Check sheet for the drawn part. Datum: minimum x, y, z corner. Units: mm. A direction names the side the tool comes from. Give positions to 0.01 mm unless a question says otherwise; leave off trailing zeros. Order: outer loops, then holes, each group sorted by start corner. A loop starts at its lowest first (then second) coordinate and runs counter-clockwise, first axis right, second up. Notation, with made-up numbers: (14, 25) - (37, 25) arc R22 ccw to (37, 45) - close; hole circle Ø10 at (77.5, 67). An arc over 180 degrees is marked (long way). Answer as a JSON object with one key per item and string values. Group by question number.
(1) Mould release check, pull along X, two halves, no side actions. Record for the marked faces 3, 4 and 5: +X half, -X half, draft (parallel to the pull), parting line (faces both ways), or undercut.
(2) Access from +Z, -Z, +X, -X, +Y, -Y to the whole of each face (thin tool, end or side, straight path). Record for the marked faces 1 and 2.
(3) Section check A-A (z = 6). Record the boundary of the cut face in (x, y).
(4) Section check B-B (y = 7.5). Record the boundary of the cut face in (x, z).
(5) Thickness scan on line 1 (X direction, y = 2, z = 5.75); line 2 (Z direction, x = 6.25, y = 11.5). Record the ranges inside material, lowest first.
(6) Depth check by flat-ended pin: pin 1 Ø4 at (x, y) = (5.5, 10.5) entering from -Z; pin 2 Ø0.6 at (x, z) = (0.5, 4.5) entering from +Y. Enter the tip coordinate at first touch or a pass-through.
(7) Section check C-C (x = 11.25). Record the boundary of the cut face in (y, z), then the cut area to 3 significant figures.
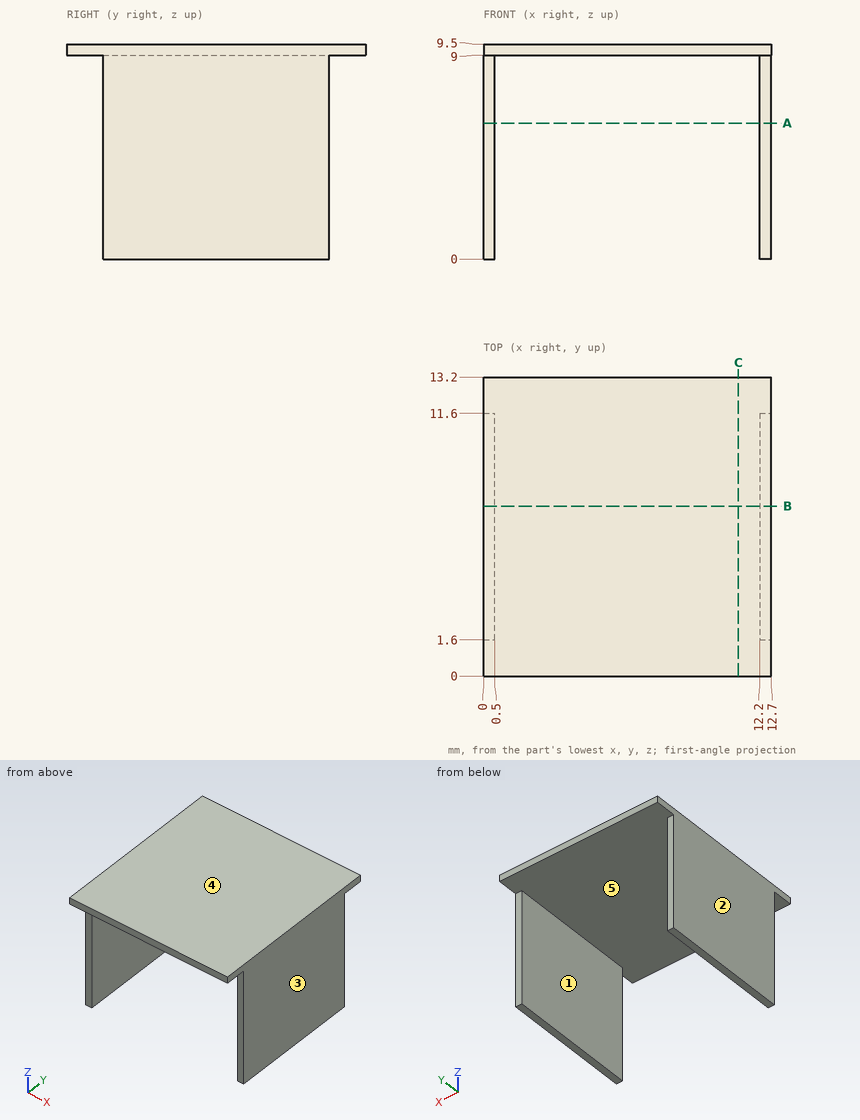
Solutions:
{
 "1": {"face 3": "+X half", "face 4": "draft", "face 5": "undercut"},
 "2": {"face 1": "-Z, +Y, -Y", "face 2": "+Z, -Z, -X, +Y, -Y"},
 "3": {"outline": "(0, 1.6) - (0.5, 1.6) - (0.5, 11.6) - (0, 11.6) - close; (12.2, 1.6) - (12.7, 1.6) - (12.7, 11.6) - (12.2, 11.6) - close"},
 "4": {"outline": "(0, 0) - (0.5, 0) - (0.5, 9) - (12.2, 9) - (12.2, 0) - (12.7, 0) - (12.7, 9.5) - (0, 9.5) - close"},
 "5": {"line 1": "x = 0 to 0.5, 12.2 to 12.7", "line 2": "z = 9 to 9.5"},
 "6": {"pin 1": "stops at z = 9", "pin 2": "stops at y = 11.6"},
 "7": {"outline": "(0, 9) - (13.2, 9) - (13.2, 9.5) - (0, 9.5) - close", "area": "6.60 mm2"}
}
